```python
from build123d import *

# Parameters (mm, degrees)
SKETCH1_R           = 1.65
SKETCH1_R_2         = 21.6
BOSS_EXTRUDE1_DEPTH = 3.6
SKETCH4_R           = 24.11
SKETCH4_R_2         = 21.7
BOSS_EXTRUDE2_DEPTH = 6.4
CHAMFER1_SIZE       = 0.2


with BuildPart() as part:
    # Sketch1 → Boss-Extrude1 (new body)
    with BuildSketch(Plane.XY):
        with BuildLine():
            Line((23.249670965, 18.073649327), (21.651772253, 16.475750615))
            ThreePointArc((21.651772253, 16.475750615), (21.3625386, 15.854117448), (21.541668543, 15.192304512))
            ThreePointArc((21.541668543, 15.192304512), (26.36, 0), (21.541668543, -15.192304512))
            ThreePointArc((21.541668543, -15.192304512), (21.3625386, -15.854117448), (21.651772253, -16.475750615))
            Line((21.651772253, -16.475750615), (23.249670965, -18.073649327))
            ThreePointArc((23.249670965, -18.073649327), (23.249670965, -23.249670965), (18.073649327, -23.249670965))
            Line((18.073649327, -23.249670965), (16.475750615, -21.651772253))
            ThreePointArc((16.475750615, -21.651772253), (15.854117448, -21.3625386), (15.192304512, -21.541668543))
            ThreePointArc((15.192304512, -21.541668543), (0, -26.36), (-15.192304512, -21.541668543))
            ThreePointArc((-15.192304512, -21.541668543), (-15.854117448, -21.3625386), (-16.475750615, -21.651772253))
            Line((-16.475750615, -21.651772253), (-18.073649327, -23.249670965))
            ThreePointArc((-18.073649327, -23.249670965), (-23.249670965, -23.249670965), (-23.249670965, -18.073649327))
            Line((-23.249670965, -18.073649327), (-21.651772253, -16.475750615))
            ThreePointArc((-21.651772253, -16.475750615), (-21.3625386, -15.854117448), (-21.541668543, -15.192304512))
            ThreePointArc((-21.541668543, -15.192304512), (-26.36, 0), (-21.541668543, 15.192304512))
            ThreePointArc((-21.541668543, 15.192304512), (-21.3625386, 15.854117448), (-21.651772253, 16.475750615))
            Line((-21.651772253, 16.475750615), (-23.249670965, 18.073649327))
            ThreePointArc((-23.249670965, 18.073649327), (-23.249670965, 23.249670965), (-18.073649327, 23.249670965))
            Line((-18.073649327, 23.249670965), (-16.475750615, 21.651772253))
            ThreePointArc((-16.475750615, 21.651772253), (-15.854117448, 21.3625386), (-15.192304512, 21.541668543))
            ThreePointArc((-15.192304512, 21.541668543), (0, 26.36), (15.192304512, 21.541668543))
            ThreePointArc((15.192304512, 21.541668543), (15.854117448, 21.3625386), (16.475750615, 21.651772253))
            Line((16.475750615, 21.651772253), (18.073649327, 23.249670965))
            ThreePointArc((18.073649327, 23.249670965), (23.249670965, 23.249670965), (23.249670965, 18.073649327))
        make_face()
        with Locations((-20.661660146, -20.661660146)):
            Circle(SKETCH1_R, mode=Mode.SUBTRACT)
        with Locations((20.661660146, -20.661660146)):
            Circle(SKETCH1_R, mode=Mode.SUBTRACT)
        Circle(SKETCH1_R_2, mode=Mode.SUBTRACT)
        with Locations(Location((20.661660146, 20.661660146, 0), (0, 0, 180))):
            Circle(SKETCH1_R, mode=Mode.SUBTRACT)
        with Locations(Location((-20.661660146, 20.661660146, 0), (0, 0, 180))):
            Circle(SKETCH1_R, mode=Mode.SUBTRACT)
    extrude(amount=BOSS_EXTRUDE1_DEPTH)

    # Sketch4 → Boss-Extrude2 (add)
    with BuildSketch(Plane.XY.offset(3.6)):
        Circle(SKETCH4_R)
        Circle(SKETCH4_R_2, mode=Mode.SUBTRACT)
    extrude(amount=BOSS_EXTRUDE2_DEPTH)

    # Sketch7 → Cut-Revolve1 (revolve, cut)
    with BuildSketch(Plane(origin=(0, 0, 0), x_dir=(1, 0, 0), z_dir=(0, 1, 0))):
        Polygon((0, -10), (0, 0), (22.5, 0), (22.5, -6), (21.7, -6.8), (21.7, -10), align=None)
    revolve(axis=Axis((0, 0, 10), (0, 0, -1)), mode=Mode.SUBTRACT)

    # Chamfer1
    chamfer1_edges = [part.edges().sort_by_distance(p)[0] for p in [
        (17.274699971, -22.450721609, 0),
        (15.854117448, -21.3625386, 0),
        (0, -26.36, 0),
        (-15.854117448, -21.3625386, 0),
        (-17.274699971, -22.450721609, 0),
        (-23.249670965, -23.249670965, 0),
        (-22.450721609, -17.274699971, 0),
        (-21.3625386, -15.854117448, 0),
        (-26.36, 0, 0),
        (-21.3625386, 15.854117448, 0),
        (-22.450721609, 17.274699971, 0),
        (-23.249670965, 23.249670965, 0),
        (-17.274699971, 22.450721609, 0),
        (-15.854117448, 21.3625386, 0),
        (0, 26.36, 0),
        (15.854117448, 21.3625386, 0),
        (17.274699971, 22.450721609, 0),
        (23.249670965, 23.249670965, 0),
        (22.450721609, 17.274699971, 0),
        (21.3625386, 15.854117448, 0),
        (26.36, 0, 0),
        (21.3625386, -15.854117448, 0),
        (22.450721609, -17.274699971, 0),
        (23.249670965, -23.249670965, 0),
        (-22.311660146, -20.661660146, 0),
        (19.011660146, -20.661660146, 0),
        (22.311660146, 20.661660146, 0),
        (-19.011660146, 20.661660146, 0),
        (-22.5, 0, 0),
    ]]
    chamfer(chamfer1_edges, length=CHAMFER1_SIZE)


solid = part.part
```
Could you check a few things on this model? Use its own coordinates, in mm. A direction names the side the tool comes from. Round coordinates to 2 decimals unless told otherwise and drop trailing zeros. Write each loop counter-clockwise with the first axis right and the second up, starting at its lowest first coordinate (ties: lowest second). Pieces come first, ordered by that corner, then holes. Notation, with made-up numbers: M 11.5,9.25 L 36.5,9.25 A28 ccw 36.5,35.25 Z; hole C -1,0 d4. An arc over 180 degrees is marked long. Answer in a Markdown table with one row per item. Add a question column.
Q1. If we mould it in two halves opening along Y, with no side actions, what happens to faces 1 (the cylindrical face through (21.88, 19.55, 1.88)), 2 (the flat face through (17.264, 22.44, 1.876)), 3 (the flat face through (0, -23, 0)), 4 (the cylindrical face through (0.23, -26.36, 1.88))? For each: +Y half, -Y half, draft (parallel to the pull), parting line (faces both ways), or undercut.
Q2. If I drill on line 1 (Y direction, x = 0.5, z = 5.75); line 2 (Y direction, x = 0, z = 7.65); line 3 (Y direction, x = 20, z = 3), over which ranges is the centre line in solid material (lowest first)? Write a range as from..to.
Q3. Imagine slicing it at A-A (y = 0). Please give me the cut outline in (x, z), then the cut area to 3 significant figures.
Q4. Imagine slicing it at C-C (z = 2.5). Give the number of separate pieces and of enclosed holes in the cut face, then the cut area to 3 significant figures.
Q5. On a 3-axis mill with a long thin cutter (end or side, diameter ignored), from which of +Z, -Z, +X, -X, +Y, -Y can I reach the whole of each face in a straight line? I mean faces 5 (the cylindrical face through (15.84, 21.36, 1.88)), 6 (the flat face through (-22.462, -17.286, 1.876)), 7 (the cylindrical face through (22.272, -9.234, 6.755)), 8 (the cylindrical face through (10.382, 19.961, 3.141)), 9 (the cylindrical face through (-15.99, 14.67, 8.38)). Say none if no direction works.
Q6. Will these pins go through, and if not, where does the flat tip stop? pin 1 Ø1 at (x, z) = (15.5, 3) entering from +Y; pin 2 Ø2 at (y, z) = (-8.5, 3.5) entering from -X; pin 3 Ø1 at (x, z) = (-17.5, 8.5) entering from +Y; pin 4 Ø5.5 at (x, y) = (20.66, -20.66) entering from -Z.
Values:
| question | item | result |
|---|---|---|
| 1 | face 1 | undercut |
| 1 | face 2 | +Y half |
| 1 | face 3 | draft |
| 1 | face 4 | -Y half |
| 2 | line 1 | -24.1..-22.49, 22.49..24.1 |
| 2 | line 2 | -24.11..-21.7, 21.7..24.11 |
| 2 | line 3 | -24.26..-22.17, -19.15..-10.31, 10.31..19.15, 22.17..24.26 |
| 3 | outline | M -26.36,0.2 L -26.16,0 L -22.7,0 L -22.5,0.2 L -22.5,6 L -21.7,6.8 L -21.7,10 L -24.11,10 L -24.11,3.6 L -26.36,3.6 Z; M 21.7,6.8 L 22.5,6 L 22.5,0.2 L 22.7,0 L 26.16,0 L 26.36,0.2 L 26.36,3.6 L 24.11,3.6 L 24.11,10 L 21.7,10 Z |
| 3 | area | 54.1 mm^2 |
| 4 | separate pieces | 1 |
| 4 | enclosed holes | 5 |
| 4 | area | 730 mm^2 |
| 5 | face 5 | +Z, -Z, +Y |
| 5 | face 6 | +Z, -Z, -X |
| 5 | face 7 | +Z |
| 5 | face 8 | -Z |
| 5 | face 9 | +Z, -Z |
| 6 | pin 1 | y = 21.68 |
| 6 | pin 2 | x = -25.27 |
| 6 | pin 3 | y = 17.1 |
| 6 | pin 4 | z = 0 |
